from build123d import *

# Parameters (mm, degrees)
SKETCH1_W            = 68
SKETCH1_H            = 27.5
BOSS_EXTRUDE1_DEPTH  = 3
FILLET1_R            = 2
SKETCH2_R            = 2.5
BOSS_EXTRUDE2_DEPTH  = 2
SKETCH4_R            = 1.05
CUT_EXTRUDE2_DEPTH   = 12
SKETCH5_W            = 5
SKETCH5_H            = 25.989939454
BOSS_EXTRUDE3_DEPTH  = 10
SKETCH6_R            = 1.55
CUT_EXTRUDE3_DEPTH   = 10
FILLET2_R            = 3
FILLET3_R            = 3
CUT_EXTRUDE4_DEPTH   = 10
FILLET4_R            = 1
FILLET4_OF_MIRROR1_R = 1


with BuildPart() as part:
    # Sketch1 → Boss-Extrude1 (new body)
    with BuildSketch(Plane(origin=(0, 0, 0), x_dir=(1, 0, 0), z_dir=(0, 1, 0))):
        with Locations((3, -0.25)):
            Rectangle(SKETCH1_W, SKETCH1_H)
    extrude(amount=BOSS_EXTRUDE1_DEPTH)

    # Fillet1
    fillet1_edges = [part.edges().sort_by_distance(p)[0] for p in [
        (-31, 1.5, -13.5),
        (37, 1.5, -13.5),
        (37, 1.5, 14),
        (-31, 1.5, 14),
    ]]
    fillet(fillet1_edges, radius=FILLET1_R)

    # Sketch2 → Boss-Extrude2 (add)
    with BuildSketch(Plane(origin=(0, 3, 0), x_dir=(1, 0, 0), z_dir=(0, 1, 0))):
        with Locations((-28, 9.5)):
            Circle(SKETCH2_R)
        with Locations((27.88, 9.5)):
            Circle(SKETCH2_R)
        with Locations((27.88, -9.55)):
            Circle(SKETCH2_R)
        with Locations((-28, -9.55)):
            Circle(SKETCH2_R)
    extrude(amount=BOSS_EXTRUDE2_DEPTH)

    # Sketch4 → Cut-Extrude2 (cut)
    with BuildSketch(Plane(origin=(0, 5, 0), x_dir=(1, 0, 0), z_dir=(0, 1, 0))):
        with Locations((-28, 9.5)):
            Circle(SKETCH4_R)
        with Locations((-28, -9.55)):
            Circle(SKETCH4_R)
        with Locations((27.88, -9.55)):
            Circle(SKETCH4_R)
        with Locations((27.88, 9.5)):
            Circle(SKETCH4_R)
    extrude(amount=-CUT_EXTRUDE2_DEPTH, mode=Mode.SUBTRACT)

    # Sketch5 → Boss-Extrude3 (add)
    with BuildSketch(Plane(origin=(0, 0, 0), x_dir=(-1, 0, 0), z_dir=(0, -1, 0))):
        with Locations((-34.5, 0)):
            Rectangle(SKETCH5_W, SKETCH5_H)
    extrude(amount=BOSS_EXTRUDE3_DEPTH)

    # Sketch6 → Cut-Extrude3 (cut)
    with BuildSketch(Plane.ZY.offset(-32)):
        with Locations((-9.5, -6)):
            Circle(SKETCH6_R)
        with Locations((9.55, -6)):
            Circle(SKETCH6_R)
    extrude(amount=-CUT_EXTRUDE3_DEPTH, mode=Mode.SUBTRACT)

    # Fillet2
    fillet2_edges = [part.edges().sort_by_distance(p)[0] for p in [
        (34.5, -10, 12.994969727),
        (34.5, -10, -12.994969727),
    ]]
    fillet(fillet2_edges, radius=FILLET2_R)

    # Fillet3
    fillet3_edges = [part.edges().sort_by_distance(p)[0] for p in [
        (32, 0, 0),
    ]]
    fillet(fillet3_edges, radius=FILLET3_R)

    # Sketch7 → Cut-Extrude4 (cut)
    with BuildSketch(Plane(origin=(0, 0, 0), x_dir=(-1, 0, 0), z_dir=(0, -1, 0))):
        Polygon((19, -9), (19, 6), (4, -9), align=None)
        Polygon((17, 9), (2, -6), (2, 9), align=None)
    cut_extrude4 = extrude(amount=-CUT_EXTRUDE4_DEPTH, mode=Mode.SUBTRACT)

    # Fillet4
    fillet4_edges = [part.edges().sort_by_distance(p)[0] for p in [
        (-2, 1.5, -9),
        (-17, 1.5, -9),
        (-2, 1.5, 6),
        (-19, 1.5, 9),
        (-4, 1.5, 9),
        (-19, 1.5, -6),
    ]]
    fillet(fillet4_edges, radius=FILLET4_R)

    # Mirror1: Cut-Extrude4 across plane
    add(cut_extrude4.mirror(Plane(origin=(0, 0, 0), x_dir=(0, 0, 1), z_dir=(1, 0, 0))), mode=Mode.SUBTRACT)

    # Fillet4 of Mirror1
    fillet4_of_mirror1_edges = [part.edges().sort_by_distance(p)[0] for p in [
        (2, 1.5, -9),
        (17, 1.5, -9),
        (2, 1.5, 6),
        (19, 1.5, 9),
        (4, 1.5, 9),
        (19, 1.5, -6),
    ]]
    fillet(fillet4_of_mirror1_edges, radius=FILLET4_OF_MIRROR1_R)


solid = part.part
Source: CAD feature listing. Evaluate the final solid. Frame: model axes, mm. A direction names the side the tool comes from. Give positions to 0.01 mm unless a question says otherwise; leave off trailing zeros. Write each loop counter-clockwise with the first axis right and the second up, starting at its lowest first coordinate (ties: lowest second). Pieces come first, ordered by that corner, then holes. Notation, with made-up numbers: (75.25, 33.25) -> (125.25, 33.25) arc R23 ccw to (125.25, 66.25) -> close; hole circle Ø8 at (62.5, 7). An arc over 180 degrees is marked (long way). Write item = value, one per line.
Q1. Cut plane D-D on x = -28. Return loops of the section in (y, z), then the cut area to 3 significant figures.
Here are the results:
outline = (0, -13.5) -> (3, -13.5) -> (3, -12) -> (5, -12) -> (5, -10.55) -> (0, -10.55) -> close; (0, -8.45) -> (5, -8.45) -> (5, -7) -> (3, -7) -> (3, 7.05) -> (5, 7.05) -> (5, 8.5) -> (0, 8.5) -> close; (0, 10.6) -> (5, 10.6) -> (5, 12.05) -> (3, 12.05) -> (3, 14) -> (0, 14) -> close
area = 81.5 mm²
Q2. First-contact query: pin 1 (2 mm diameter, centred on y = -7.5, z = 5, fed in from -X); pin 2 (3 mm diameter, centred on x = 1, z = -7.5, fed in from +Y); pin 3 (2 mm diameter, centred on x = 33.5, y = -2.5, fed in from -Z). Flat tips, straight axial feed; report the tip coordinate or a pass-through.
Here are the results:
pin_1 = 32
pin_2 = 3
pin_3 = -12.99
Q3. Reachability of faces 4 (the face through (-28, 5, 11)), 5 (the face through (-12, 1, 1)), 6 (the face through (36.43, 1.52, -12.9)), 7 (the face through (-28.54, 3.99, -7.06)), 8 (the face through (34, -3, -12.995)) from +Z, -Z, +X, -X, +Y, -Y: full face, straight path, thin tool, end or side. Return the list, or none.
Here are the results:
face_4 = +Z, -Z, +X, -X, +Y
face_5 = +Y, -Y
face_6 = -Z, +X, +Y
face_7 = +Y
face_8 = -Z, +X, -X, -Y
Q4. Cut plane C-C on z = 1.25. Return loops of the section in (x, y), then the cut area to 3 significant figures.
Here are the results:
outline = (-31, 0) -> (-19, 0) -> (-19, 3) -> (-31, 3) -> close; (-11.75, 0) -> (-6.75, 0) -> (-6.75, 3) -> (-11.75, 3) -> close; (-2, 0) -> (2, 0) -> (2, 3) -> (-2, 3) -> close; (6.75, 0) -> (11.75, 0) -> (11.75, 3) -> (6.75, 3) -> close; (19, 0) -> (29, 0) arc R3 cw to (32, -3) -> (32, -10) -> (37, -10) -> (37, 3) -> (19, 3) -> close
area = 184 mm²
Q5. Mould query, pull axis X, two halves, no side actions, for faces 1 (the face through (32, -6, 0)), 2 (the face through (30.265, 3.986, 8.799)), 3 (the face through (34.47, -9.1, 12.14)). Classes: +X half, -X half, draft (parallel to the pull), parting line (faces both ways), or undercut.
Here are the results:
face_1 = -X half
face_2 = undercut
face_3 = draft
Q6. Line query: line 1 (Z direction, x = 27.88, y = 1.8); line 2 (X direction, y = 2.6, z = 9.55); line 3 (Z direction, x = -28, y = 3.7). Output: solid intervals per line, ascending. Write a range as from..to.
Here are the results:
line_1 = -13.5..-10.55, -8.45..8.5, 10.6..14
line_2 = -31..-29.05, -26.95..26.83, 28.93..37
line_3 = -12..-10.55, -8.45..-7, 7.05..8.5, 10.6..12.05
Q7. Cut plane B-B on x = -8. Return loops of the section in (y, z), then the cut area to 3 significant figures.
Here are the results:
outline = (0, -13.5) -> (3, -13.5) -> (3, -9) -> (0, -9) -> close; (0, 0) -> (3, 0) -> (3, 5) -> (0, 5) -> close; (0, 9) -> (3, 9) -> (3, 14) -> (0, 14) -> close
area = 43.5 mm²
Q8. Cut plane A-A on y = -6. Return loops of the section in (x, z), then the cut area to 3 significant figures.
Here are the results:
outline = (32, -12.99) -> (37, -12.99) -> (37, -11.05) -> (32, -11.05) -> close; (32, -7.95) -> (37, -7.95) -> (37, 8) -> (32, 8) -> close; (32, 11.1) -> (37, 11.1) -> (37, 12.99) -> (32, 12.99) -> close
area = 98.9 mm²
